Model file for the job. Use its own axes, mm. Face numbers are marked on the shaded views. Give positions to 0.01 mm unless a question says otherwise; leave off trailing zeros. Write each loop counter-clockwise with the first axis right and the second up, starting at its lowest first coordinate (ties: lowest second). Pieces come first, ordered by that corner, then holes.
```python
from build123d import *

# Parameters (mm, degrees)
F0_W     = 34
F0_H     = 22
F1_DEPTH = 4
F2_SIZE  = 2
F3_W     = 30
F3_H     = 15
F4_DEPTH = 1.5
F5_R     = 1.169255
F5_R_2   = 1.258596
F6_DEPTH = 25


with BuildPart() as f1:
    # F0 (on Top) → F1 (new body)
    with BuildSketch(Plane.XY):
        Rectangle(F0_W, F0_H)
    extrude(amount=F1_DEPTH)

    # F2
    f2_edges = [f1.edges().sort_by_distance(p)[0] for p in [
        (-17, 0, 0),
        (17, 0, 0),
        (0, 11, 0),
        (0, -11, 0),
    ]]
    chamfer(f2_edges, length=F2_SIZE)

    # F3 (on face) → F4 (cut)
    with BuildSketch(Plane.XY.offset(4)):
        Rectangle(F3_W, F3_H)
    extrude(amount=-F4_DEPTH, mode=Mode.SUBTRACT)

    # F5 (on face) → F6 (cut)
    with BuildSketch(Plane.XY.offset(2.5)):
        with Locations((-12.872203, 5.703713)):
            Circle(F5_R)
        with Locations((12.584788, 5.37942)):
            Circle(F5_R_2)
    extrude(amount=-F6_DEPTH, mode=Mode.SUBTRACT)


solid = f1.part
```
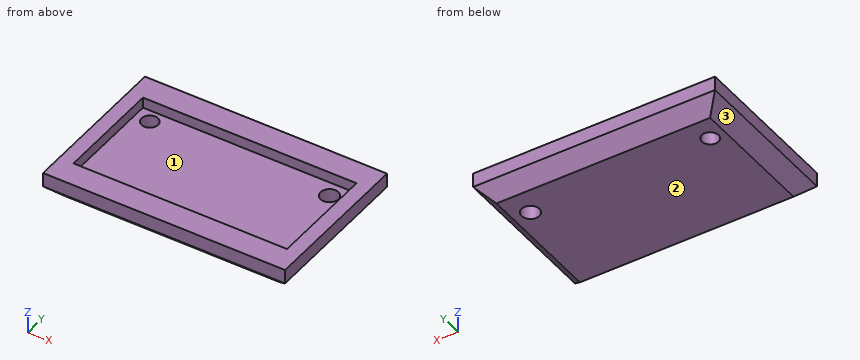
1. Slice it at A-A, the plane z = 3.4. Write the cut outline in (x, y).
Calculated:
outline: (-17, -11) - (17, -11) - (17, 11) - (-17, 11) - close; hole (-15, -7.5) - (15, -7.5) - (15, 7.5) - (-15, 7.5) - close
2. Pull direction X, two halves, no side cores. Call the marked faces 1, 2 and 3: +X half, -X half, draft (parallel to the pull), parting line (faces both ways), or undercut.
Calculated:
face 1: undercut
face 2: draft
face 3: -X half
3. Pin check, flat tip, straight feed: P1, Ø10, axis at x = 3.5, y = 1, coming from the +Z side. Stop position of the tip, or through.
Calculated:
P1: stops at z = 2.5
4. Slice it at D-D, the plane x = -13. Write the cut outline in (y, z), and give its area (3 significant figures).
Calculated:
outline: (-11, 2) - (-9, 0) - (4.54, 0) - (4.54, 2.5) - (-7.5, 2.5) - (-7.5, 4) - (-11, 4) - close; (6.87, 0) - (9, 0) - (11, 2) - (11, 4) - (7.5, 4) - (7.5, 2.5) - (6.87, 2.5) - close
area: 55.7 mm2
5. Slice it at C-C, the plane y = -6.5. Write the cut outline in (x, z), and give its area (3 significant figures).
Calculated:
outline: (-17, 2) - (-15, 0) - (15, 0) - (17, 2) - (17, 4) - (15, 4) - (15, 2.5) - (-15, 2.5) - (-15, 4) - (-17, 4) - close
area: 87.0 mm2
6. Probe probe 1 along Y at (x, z) = (-5, 2.8); probe 2 along X at (y, z) = (3.5, 3); probe 3 along X at (y, z) = (5, 0.85). List the from-to ranges inside material, lowest first.
Calculated:
probe 1: y = -11 to -7.5, 7.5 to 11
probe 2: x = -17 to -15, 15 to 17
probe 3: x = -15.85 to -13.81, -11.94 to 11.38, 13.78 to 15.85
7. Slice it at B-B, the plane x = 15.5. Write the cut outline in (y, z), and give its area (4 significant figures).
Calculated:
outline: (-11, 2) - (-9.5, 0.5) - (9.5, 0.5) - (11, 2) - (11, 4) - (-11, 4) - close
area: 74.75 mm2
